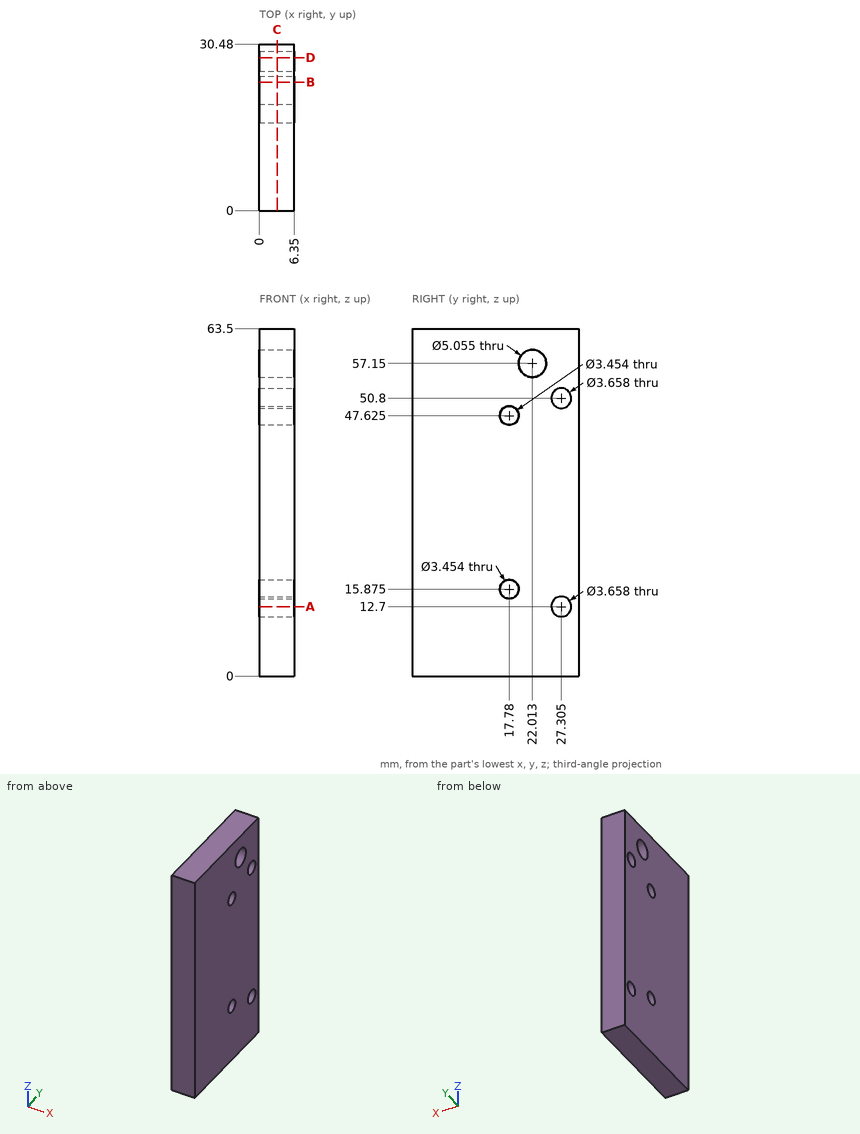
Input: dimensioned drawing with shaded views. Units: mm. Origin: part minimum x, y, z. Give positions to 0.01 mm unless a question says otherwise; leave off trailing zeros. Write each loop counter-clockwise with the first axis right and the second up, starting at its lowest first coordinate (ties: lowest second). Pieces come first, ordered by that corner, then holes. Notation, with made-up numbers: M 45.5,54.5 L 102.5,54.5 A23 ccw 102.5,79.5 Z; hole C 77,-9.5 d7. An arc over 180 degrees is marked long. Return JSON: item names as keys, results as strings. Group by question number.
1) Material intervals for line 1 along Z through (x, y) = (4.25, 17.78); line 2 along Y through (x, z) = (2.75, 57); line 3 along Y through (x, z) = (2.5, 50.8), sorted ascending. Write a range as [from, to].
2) Cut plane A-A, the plane z = 12.7. Output: boundary loops of the cut face in (x, y), plus the area to 3 significant figures.
3) Cut plane B-B, the plane y = 23.5. Output: boundary loops of the cut face in (x, z).
4) Cut plane D-D, the plane y = 28. Output: boundary loops of the cut face in (x, z).
5) Cut plane C-C, the plane x = 3.25. Give the number of separate pieces and of enclosed holes in the cut face, plus the area to 3 significant figures.
6) Pin query (flat end, axial travel): P1, Ø3.5, axis at y = 27.305, z = 50.8, coming from the +X side. Return the tip coordinate at first contact, or that it passes through.
Recorded:
{
 "1": {"line 1": "z = [0, 14.15], [17.6, 45.9], [49.35, 63.5]", "line 2": "y = [0, 19.49], [24.54, 30.48]", "line 3": "y = [0, 25.48], [29.13, 30.48]"},
 "2": {"outline": "M 0,0 L 6.35,0 L 6.35,25.48 L 0,25.48 Z; M 0,29.13 L 6.35,29.13 L 6.35,30.48 L 0,30.48 Z", "area": "170 mm²"},
 "3": {"outline": "M 0,0 L 6.35,0 L 6.35,55.11 L 0,55.11 Z; M 0,59.19 L 6.35,59.19 L 6.35,63.5 L 0,63.5 Z"},
 "4": {"outline": "M 0,0 L 6.35,0 L 6.35,11.01 L 0,11.01 Z; M 0,14.39 L 6.35,14.39 L 6.35,49.11 L 0,49.11 Z; M 0,52.49 L 6.35,52.49 L 6.35,63.5 L 0,63.5 Z"},
 "5": {"separate pieces": "1", "enclosed holes": "5", "area": "1,880 mm²"},
 "6": {"P1": "passes through"}
}
